Geometry: final body of the model. Coordinates: model frame, mm. A direction names the side the tool comes from. Give positions to 0.01 mm unless a question says otherwise; leave off trailing zeros. Write each loop counter-clockwise with the first axis right and the second up, starting at its lowest first coordinate (ties: lowest second). Pieces come first, ordered by that corner, then holes. Notation, with made-up numbers: M 49,69.5 L 90,69.5 A12 cw 90,92.5 Z; hole C -32,19 d5. An arc over 180 degrees is marked long. Use a Markdown table: item, result. Add a question column.
1) Section A-A on z = 10. Return the cut outline in (x, y).
2) Section D-D on x = 11. Return the cut outline in (y, z).
3) Line query: line 1 (Z direction, x = -0.95, y = 20); line 2 (Y direction, x = 10, z = 5); line 3 (Z direction, x = 10.5, y = -13.8). Output: solid intervals per line, ascending.
4) Section B-B on y = 20. Return the cut outline in (x, z).
5) Pin query (flat end, axial travel): pin 1 (5 mm diameter, centred on y = -10, z = 5, fed in from +X); pin 2 (1 mm diameter, centred on x = 12, y = -2.5, fed in from +Z); pin 3 (12 mm diameter, centred on y = 3, z = 7.5, fed in from +X); pin 4 (2.5 mm diameter, centred on x = 10.5, y = 14, fed in from +Z). Return the tip coordinate at first contact, or that it passes through.
6) Section C-C on z = 0. Return the cut outline in (x, y).
7) Draft query along Z for faces 4 (the cylindrical face through (7.9, 12.9, 0)), 5 (the flat face through (0, 0, 0)), 6 (the cylindrical face through (-1.5, 17.5, -19.9)), 7 (the flat face through (-1, 0, -25)). Return one class per face: +Z half, -Z half, draft (parallel to the pull), parting line (faces both ways), or undercut.
8) Set-up query: faces 1 (the flat face through (12, -14, 10.9)), 2 (the flat face through (8, -14, 2)), 3 (the flat face through (0, 14, 0)). Return all of +Z, -Z, +X, -X, +Y, -Y with unobstructed straight access to the full face (end or side cutting, diameter ignored); none if empty.
```python
from build123d import *

# Parameters (mm, degrees)
F0_R     = 0.9
F1_DEPTH = 16
F2_W     = 8
F2_H     = 16.8
F3_DEPTH = 5
F4_W     = 50
F4_H     = 50
F4_R     = 2.5
F5_DEPTH = 3


with BuildPart() as f1:
    # F0 (on Right) → F1 (new body)
    with BuildSketch(Plane.YZ):
        Polygon((-16.1, 10.9), (-16.1, 5.9), (-16.1, -5.9), (-16.1, -10.9), (16.1, -10.9), (16.1, -5.9), (16.1, 5.9), (16.1, 10.9), (11.4, 10.9), (11.4, 5.9), (11.4, -5.9), (11.4, -6.4), (-11.4, -6.4), (-11.4, -5.9), (-11.4, 5.9), (-11.4, 10.9), align=None)
        with Locations((-13.8, 0)):
            Circle(F0_R, mode=Mode.SUBTRACT)
        with Locations((13.8, 0)):
            Circle(F0_R, mode=Mode.SUBTRACT)
    extrude(amount=F1_DEPTH)

    # F2 (on face) → F3 (cut)
    with BuildSketch(Plane.XZ.offset(16.1)):
        with Locations((4, 2.5)):
            Rectangle(F2_W, F2_H)
    extrude(amount=-F3_DEPTH, mode=Mode.SUBTRACT)

    # F4 (on face) → F5 (join)
    with BuildSketch(Plane.YZ):
        Rectangle(F4_W, F4_H)
        with Locations((-20, -20)):
            Circle(F4_R, mode=Mode.SUBTRACT)
        with Locations((20, -20)):
            Circle(F4_R, mode=Mode.SUBTRACT)
        with Locations((-20, 20)):
            Circle(F4_R, mode=Mode.SUBTRACT)
        with Locations((20, 20)):
            Circle(F4_R, mode=Mode.SUBTRACT)
    extrude(amount=-F5_DEPTH)


solid = f1.part
```
Found:
| question | item | result |
|---|---|---|
| 1 | outline | M -3,-25 L 0,-25 L 0,11.4 L 16,11.4 L 16,16.1 L 0,16.1 L 0,25 L -3,25 Z; M 8,-16.1 L 16,-16.1 L 16,-11.4 L 8,-11.4 Z |
| 2 | outline | M -16.1,-10.9 L 16.1,-10.9 L 16.1,10.9 L 11.4,10.9 L 11.4,-6.4 L -11.4,-6.4 L -11.4,10.9 L -16.1,10.9 Z; hole C -13.8,0 d1.8; hole C 13.8,0 d1.8 |
| 3 | line 1 | -25 to -22.5, -17.5 to 17.5, 22.5 to 25 |
| 3 | line 2 | -16.1 to -11.4, 11.4 to 16.1 |
| 3 | line 3 | -10.9 to -0.9, 0.9 to 10.9 |
| 4 | outline | M -3,-25 L 0,-25 L 0,-22.5 L -3,-22.5 Z; M -3,-17.5 L 0,-17.5 L 0,17.5 L -3,17.5 Z; M -3,22.5 L 0,22.5 L 0,25 L -3,25 Z |
| 5 | pin 1 | x = 16 |
| 5 | pin 2 | z = -6.4 |
| 5 | pin 3 | x = 0 |
| 5 | pin 4 | z = 10.9 |
| 6 | outline | M -3,-25 L 0,-25 L 0,11.4 L 16,11.4 L 16,12.9 L 0,12.9 L 0,14.7 L 16,14.7 L 16,16.1 L 0,16.1 L 0,25 L -3,25 Z; M 8,-16.1 L 16,-16.1 L 16,-14.7 L 8,-14.7 Z; M 8,-12.9 L 16,-12.9 L 16,-11.4 L 8,-11.4 Z |
| 7 | face 4 | undercut |
| 7 | face 5 | draft |
| 7 | face 6 | undercut |
| 7 | face 7 | -Z half |
| 8 | face 1 | +Z, +X, +Y, -Y |
| 8 | face 2 | +Z, -Y |
| 8 | face 3 | +X |
